Work out the finished part from the listing and answer in its coordinate system (mm). Face numbers are marked on the shaded views. Round coordinates to 2 decimals unless told otherwise and drop trailing zeros. Write each loop counter-clockwise with the first axis right and the second up, starting at its lowest first coordinate (ties: lowest second). Pieces come first, ordered by that corner, then holes.
1. Find section A-A (x = 5). Write down the section's boundary in (y, z).
2. Find section C-C (z = 0.8). Write down the section's boundary in (x, y).
3. Straight lines are drawn through the part: probe 1 along Y at (x, z) = (5, -1.3); probe 2 along Y at (x, z) = (6.5, -1.7); probe 3 along X at (y, z) = (-1, 2.2). For each, find the intervals that lie inside material, in ascending order.
4. Find section B-B (y = 0). Write down the section's boundary in (x, z), and give its area (3 significant figures).
5. Determine the mould class of the marked faces 1, 2 and 3 for opening direction Y: pulls with the +Y half, pulls with the -Y half, needs draft (parallel to the pull), parting line crosses it, or undercut.
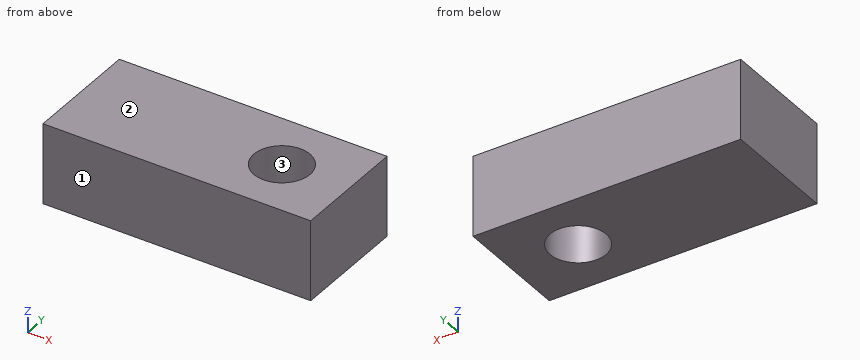
```python
from build123d import *

# Parameters (mm, degrees)
SKETCH_1_W      = 20
SKETCH_1_H      = 8.7
SKETCH_1_R      = 2.1
EXTRUDE_1_DEPTH = 3


with BuildPart() as part:
    # 草图1 → 凸台-拉伸1 (new, symmetric)
    with BuildSketch(Plane.XY):
        Rectangle(SKETCH_1_W, SKETCH_1_H)
        with Locations((5, 0)):
            Circle(SKETCH_1_R, mode=Mode.SUBTRACT)
    extrude(amount=EXTRUDE_1_DEPTH, both=True)


solid = part.part
```
Worked answers:
1. outline: (-4.35, -3) - (-2.1, -3) - (-2.1, 3) - (-4.35, 3) - close; (2.1, -3) - (4.35, -3) - (4.35, 3) - (2.1, 3) - close
2. outline: (-10, -4.35) - (10, -4.35) - (10, 4.35) - (-10, 4.35) - close; hole circle Ø4.2 at (5, 0)
3. probe 1: y = -4.35 to -2.1, 2.1 to 4.35
3. probe 2: y = -4.35 to -1.47, 1.47 to 4.35
3. probe 3: x = -10 to 3.15, 6.85 to 10
4. outline: (-10, -3) - (2.9, -3) - (2.9, 3) - (-10, 3) - close; (7.1, -3) - (10, -3) - (10, 3) - (7.1, 3) - close
4. area: 94.8 mm2
5. face 1: pulls with the -Y half
5. face 2: needs draft
5. face 3: undercut
